from build123d import *

# Parameters (mm, degrees)
ESQUISSE3_R        = 1.35255
ESQUISSE3_R_2      = 2.7051
ESQUISSE3_R_3      = 1.55
ESQUISSE3_R_4      = 4
BOSS_EXTRU_2_DEPTH = 3


with BuildPart() as part:
    # Esquisse3 → Boss.-Extru.2 (new body)
    with BuildSketch(Plane(origin=(0, 0, 0), x_dir=(0, 0, -1), z_dir=(1, 0, 0))):
        with BuildLine():
            Line((-40.60825, -16.144875), (-40.60825, -16.348305132))
            add(Edge.make_bspline(
                [(-40.60825, -16.348305132), (-40.365634485, -16.661193605), (-40.112338127, -16.96547542), (-39.63020507, -17.593748723), (-39.400688032, -17.917191992), (-38.719045939, -18.893089111), (-38.271947044, -19.549593057), (-37.338540998, -20.831006808), (-36.855460104, -21.458516341), (-36.059725811, -22.342477591), (-35.781944124, -22.627029047), (-35.202868212, -23.17718548), (-34.900674383, -23.443503751), (-33.971943166, -24.212706181), (-33.324405882, -24.685383849), (-32.010805282, -25.604549776), (-31.348089528, -26.055770333), (-30.303090708, -26.660610546), (-29.948270215, -26.848696892), (-29.222483721, -27.184971005), (-28.851412004, -27.333773538), (-28.083597976, -27.570691368), (-27.685315555, -27.657976057), (-27.090666934, -27.715403346), (-26.891908645, -27.722631025), (-26.592836888, -27.712936491), (-26.492990431, -27.706278992), (-26.292963936, -27.685632014), (-26.192732932, -27.670522326), (-26.092449031, -27.65425)],
                knots=[0, 0, 0, 0, 0.0625, 0.0625, 0.125, 0.125, 0.25, 0.25, 0.375, 0.375, 0.4375, 0.4375, 0.5, 0.5, 0.625, 0.625, 0.75, 0.75, 0.8125, 0.8125, 0.875, 0.875, 0.9375, 0.9375, 0.96875, 0.96875, 0.984375, 0.984375, 1, 1, 1, 1], degree=3))
            Line((-26.092449031, -27.65425), (-26.092449031, -90))
            ThreePointArc((-26.092449031, -90), (-2.31531669, -116.14013034), (25.954024412, -94.93864949))
            Line((25.954024412, -94.93864949), (25.954024412, -27.65425))
            add(Edge.make_bspline(
                [(25.954024412, -27.65425), (27.179118802, -27.419536533), (28.353377808, -27.051803075), (30.05705383, -26.34918771), (30.615126485, -26.089288473), (31.712904721, -25.521429223), (32.254485024, -25.212118815), (33.827204106, -24.230350536), (34.814025463, -23.502087852), (36.672007358, -21.907218093), (37.543320305, -21.040793316), (38.751902771, -19.623473398), (39.134714509, -19.134962989), (39.851014333, -18.131439591), (40.185535135, -17.615291382), (40.801362362, -16.550595558), (41.082635497, -16.002027673), (41.457015911, -15.150237789), (41.574249194, -14.86042264), (41.789713906, -14.277065554), (41.888049248, -13.98351322), (42.334688534, -12.506770959), (42.546239761, -11.296312151), (42.717568356, -9.451511475), (42.750611649, -8.83067761), (42.772859866, -7.900507946), (42.775360474, -7.590422151), (42.77555993, -6.970221998), (42.772087252, -6.66010067), (42.772087252, -6.35)],
                knots=[0, 0, 0, 0, 0.125, 0.125, 0.1875, 0.1875, 0.25, 0.25, 0.375, 0.375, 0.5, 0.5, 0.5625, 0.5625, 0.625, 0.625, 0.6875, 0.6875, 0.71875, 0.71875, 0.75, 0.75, 0.875, 0.875, 0.9375, 0.9375, 0.96875, 0.96875, 1, 1, 1, 1], degree=3))
            add(Edge.make_bspline(
                [(42.772087252, -6.35), (42.772087252, -5.874878454), (42.783792207, -5.398095979), (42.789657917, -4.447020546), (42.781867467, -3.973004463), (42.672546396, -2.563152451), (42.499179213, -1.637510108), (42.106282017, -0.267897459), (41.954068536, 0.185625042), (41.614819435, 1.087728793), (41.430081297, 1.530283034), (40.844911495, 2.839259084), (40.416604561, 3.689518781), (39.046783283, 6.190525131), (38.013123304, 7.787251584), (36.291657446, 10.082106977), (35.688509547, 10.830664164), (34.43654182, 12.281738953), (33.786199883, 12.985690235), (33.112075, 13.668565083)],
                knots=[0, 0, 0, 0, 0.0625, 0.0625, 0.125, 0.125, 0.25, 0.25, 0.3125, 0.3125, 0.375, 0.375, 0.5, 0.5, 0.75, 0.75, 0.875, 0.875, 1, 1, 1, 1], degree=3))
            add(Edge.make_bspline(
                [(33.112075, 13.668565083), (32.332207955, 14.539101946), (31.435060987, 15.277734234)],
                knots=[0, 0, 0, 1, 1, 1], degree=2))
            add(Edge.make_bspline(
                [(31.435060987, 15.277734234), (30.299691041, 16.309376592), (29.113704516, 17.275445235), (26.646604831, 19.084346085), (25.360475951, 19.928267183), (21.432297769, 22.265681686), (18.70167828, 23.563722979), (14.477833082, 25.213127628), (13.049229105, 25.71486416), (10.864398428, 26.369911185), (10.129061703, 26.571832136), (8.64156399, 26.936524394), (7.890831572, 27.098844789), (5.637990782, 27.512412208), (4.127431428, 27.693727696), (2.225306731, 27.768676851), (1.844136038, 27.775542931), (1.080940786, 27.779973661), (0.698904769, 27.777413484), (-0.446346689, 27.779064109), (-1.208874123, 27.797823926), (-2.732682239, 27.815308111), (-3.492085471, 27.806304753), (-5.004084105, 27.739990771), (-5.756994671, 27.684916502), (-8.006157922, 27.451797552), (-9.492662784, 27.204583891), (-11.701987236, 26.688775277), (-12.434852331, 26.491461598), (-13.894254142, 26.051929085), (-14.622118919, 25.807493497), (-16.765417144, 25.01223388), (-18.151500369, 24.400517874), (-20.847821735, 23.032525232), (-22.158708475, 22.277484827), (-24.716496252, 20.645447351), (-25.966430559, 19.7652326), (-28.39125747, 17.919703458), (-29.567431908, 16.954258357), (-31.287557173, 15.454109034), (-31.85380584, 14.945666112), (-32.972832423, 13.91291508), (-33.52577931, 13.388805977), (-34.066096443, 12.849822171)],
                knots=[0, 0, 0, 0, 0.0625, 0.0625, 0.125, 0.125, 0.25, 0.25, 0.3125, 0.3125, 0.34375, 0.34375, 0.375, 0.375, 0.4375, 0.4375, 0.453125, 0.453125, 0.46875, 0.46875, 0.5, 0.5, 0.53125, 0.53125, 0.5625, 0.5625, 0.625, 0.625, 0.65625, 0.65625, 0.6875, 0.6875, 0.75, 0.75, 0.8125, 0.8125, 0.875, 0.875, 0.9375, 0.9375, 0.96875, 0.96875, 1, 1, 1, 1], degree=3))
            add(Edge.make_bspline(
                [(-34.066096443, 12.849822171), (-35.159801618, 11.692162737), (-36.251081621, 10.53740284), (-37.166580532, 9.404947171)],
                knots=[0, 0, 0, 0, 1, 1, 1, 1], degree=3))
            ThreePointArc((-37.166580532, 9.404947171), (-37.363014685, 9.160281042), (-37.557796616, 8.914297524))
            add(Edge.make_bspline(
                [(-37.557796616, 8.914297524), (-38.142933539, 8.170182683), (-38.709522845, 7.412667282), (-39.741912272, 5.824816801), (-40.203133529, 4.998794666), (-40.60825, 4.142494902)],
                knots=[0, 0, 0, 0, 0.5, 0.5, 1, 1, 1, 1], degree=3))
            Line((-40.60825, 4.142494902), (-40.60825, -12.7))
            Line((-40.60825, -12.7), (-40.60825, -16.144875))
        make_face()
        with Locations((-16.9799, -14.9225)):
            Circle(ESQUISSE3_R, mode=Mode.SUBTRACT)
        with Locations((0.1651, -18.2245)):
            Circle(ESQUISSE3_R_2, mode=Mode.SUBTRACT)
        with Locations((17.3101, -14.9225)):
            Circle(ESQUISSE3_R, mode=Mode.SUBTRACT)
        with Locations((0.1651, 6.103472306)):
            Circle(ESQUISSE3_R, mode=Mode.SUBTRACT)
        with Locations((0.1651, -103.128774516)):
            Circle(ESQUISSE3_R_3, mode=Mode.SUBTRACT)
        with Locations((-12.956172959, -90)):
            Circle(ESQUISSE3_R_3, mode=Mode.SUBTRACT)
        with Locations((0.1651, -76.853281608)):
            Circle(ESQUISSE3_R_3, mode=Mode.SUBTRACT)
        with Locations((13.293874516, -90)):
            Circle(ESQUISSE3_R_3, mode=Mode.SUBTRACT)
        with Locations((0.1651, -90)):
            Circle(ESQUISSE3_R_4, mode=Mode.SUBTRACT)
        with BuildLine():
            Line((-6.1849, 6.103472306), (-6.1849, 11.646916554))
            ThreePointArc((-6.1849, 11.646916554), (-15.726599278, 6.86795928), (-22.463125, -1.408614826))
            Line((-22.463125, -1.408614826), (-22.848998606, -8.5725))
            Line((-22.848998606, -8.5725), (-16.9799, -8.5725))
            ThreePointArc((-16.9799, -8.5725), (-14.843492837, -8.942678562), (-12.956172959, -10.010054509))
            Line((-12.956172959, -10.010054509), (-17.532119892, -76.570733548))
            ThreePointArc((-17.532119892, -76.570733548), (-12.922094173, -82.243210377), (-7.579161123, -77.254984547))
            Line((-7.579161123, -77.254984547), (-3.118194312, -12.366780117))
            ThreePointArc((-3.118194312, -12.366780117), (3.559593485, -12.430510205), (6.880225, -18.2245))
            Line((6.880225, -18.2245), (6.880225, -21.669375))
            Line((6.880225, -21.669375), (10.9601, -21.669375))
            Line((10.9601, -21.669375), (10.9601, -14.9225))
            ThreePointArc((10.9601, -14.9225), (12.819971939, -10.432371939), (17.3101, -8.5725))
            Line((17.3101, -8.5725), (23.12590424, -8.5725))
            Line((23.12590424, -8.5725), (22.793325, -1.408614826))
            ThreePointArc((22.793325, -1.408614826), (16.056799278, 6.86795928), (6.5151, 11.646916554))
            Line((6.5151, 11.646916554), (6.5151, 6.103472306))
            ThreePointArc((6.5151, 6.103472306), (0.1651, -0.246527694), (-6.1849, 6.103472306))
        make_face(mode=Mode.SUBTRACT)
    extrude(amount=BOSS_EXTRU_2_DEPTH)


solid = part.part
Could you check a few things on this model? Use its own coordinates, in mm. A direction names the side the tool comes from. Coordinates: 2 decimals unless noted, no trailing zeros. Order: outer loops, then holes, each group sorted by start corner. A loop starts at its lowest first (then second) coordinate and runs counter-clockwise, first axis right, second up. Notation, with made-up numbers: (87.25, 5) -> (95.25, 5) arc R24 cw to (95.25, 39) -> close; hole circle Ø6 at (-11, 17). An arc over 180 degrees is marked (long way). One line per item, written item: value. Start each with the question number.
1) If I drill on L1, parallel to Z at x = 2.65, y = -76; L2, parallel to Y at x = 1.75, z = -2.5; L3, parallel to Y at x = 1.9, z = 1.5, over which ranges is the centre line in solid material (lowest first)? Write a range as [from, to].
2) Which directions (+Z, -Z, +X, -X, +Y, -Y) give clear straight access to the entire face, cutting with the end or side of a thin tool? Please do faces 1 (the flat face through (0, -43, -1)), 2 (the flat face through (1.48, -5.04, -22.96)).
3) Imagine slicing it at A-A on y = -41. List the corners of the cut face in (x, z) for me, plus the area to 3 significant figures.
4) Imagine slicing it at C-C on y = -97. List the corners of the cut face in (x, z) for me, plus the area to 3 significant figures.
5) We'd pull the mould along Y, two halves only. Please class faces 3 (the cylindrical face through (1.479, -116.083, 2.855)), 4 (the flat face through (1, -6, 40.608)), 5 (the cylindrical face through (1.479, -75.316, 0.037)): +Y half, -Y half, draft (parallel to the pull), parting line (faces both ways), or undercut.
6) I'm going to push flat-ended pins straight in: pin 1 (1.5 mm diameter, centred on x = 0.5, y = -39.5, fed in from -Z); pin 2 (1.5 mm diameter, centred on x = 1.5, z = -20.5, fed in from +Y); pin 3 (2.5 mm diameter, centred on y = 6.1, z = -0.17, fed in from -X); pin 4 (0.9 mm diameter, centred on x = 2, y = -18.5, fed in from +Z). Where does each tip first touch, or does it pass through?
7) Imagine slicing it at B-B on x = 0.85. Count the separate pieces of the cut face and the enclosed holes in it, plus the area to 3 significant figures.
Answer list:
1. L1: z = [-25.95, -1.46], [1.13, 7.49], [17.49, 26.09]
1. L2: y = [-116.15, -93.25], [-86.75, -19.59], [-16.86, -11.93], [0.2, 27.76]
1. L3: y = [-116.2, -93.64], [-86.36, -20.36], [-16.09, -11.72], [-0.02, 27.8]
2. face 1: +Z, -Z, -X, +Y, -Y
2. face 2: +X, -X
3. outline: (0, -25.95) -> (3, -25.95) -> (3, 5.09) -> (0, 5.09) -> close; (0, 15.09) -> (3, 15.09) -> (3, 26.09) -> (0, 26.09) -> close
3. area: 126 mm2
4. outline: (0, -25.47) -> (3, -25.47) -> (3, 25.14) -> (0, 25.14) -> close
4. area: 152 mm2
5. face 3: -Y half
5. face 4: draft
5. face 5: undercut
6. pin 1: stops at z = -25.95
6. pin 2: stops at y = 23
6. pin 3: passes through
6. pin 4: stops at z = 39.31
7. separate pieces: 1
7. enclosed holes: 10
7. area: 6,600 mm2
